Verification items for the finished model (mm, model axes). A direction names the side the tool comes from. Coordinates: 2 decimals unless noted, no trailing zeros. Order: outer loops, then holes, each group sorted by start corner. A loop starts at its lowest first (then second) coordinate and runs counter-clockwise, first axis right, second up. Notation, with made-up numbers: (81.5, 26.25) -> (105.5, 26.25) arc R14 ccw to (105.5, 35.25) -> close; hole circle Ø2 at (71, 81.25). An arc over 180 degrees is marked (long way). Write each question's results on one line, items separated by ' | '. Start each with the question number.
(1) Thickness scan on probe 1 along Y at (x, z) = (-5, 0); probe 2 along X at (y, z) = (2.35, 10); probe 3 along X at (y, z) = (-2, 1). Record the ranges inside material, lowest first. Write a range as [from, to].
(2) Cross-section at A-A on z = 10. Enter the section's corners in (x, y).
(3) Cross-section at D-D on y = -6.5. Enter the section's corners in (x, z), and give its area (3 significant figures).
(4) Draft check along X on faces 4 (the cylindrical face through (-9.51, 1.97, 9.87)), 5 (the cylindrical face through (-12.93, 2.03, -12.4)), 6 (the cylindrical face through (5, -8, 4)). Enter one of: +X half, -X half, draft (parallel to the pull), parting line (faces both ways), or undercut.
(5) Cross-section at C-C on y = 1. Enter the section's corners in (x, z), and give its area (3 significant figures).
(6) Set-up check for faces 1 (the flat face through (5, -2, 5)), 2 (the flat face through (7.5, -2.7, -0.1)), 3 (the flat face through (-5, -2, -5)): record each of +Z, -Z, +X, -X, +Y, -Y from which the full face is reachable in a straight line by a thin tool's end or side.
(7) Go/stop test with flat-tipped pins: pin 1 (8 mm diameter, centred on y = -4.5, z = -1.5, fed in from +X); pin 2 (3 mm diameter, centred on y = -3, z = -1, fed in from -X); pin 3 (1.5 mm diameter, centred on x = -10.5, y = -2.5, fed in from -Z); pin 4 (4 mm diameter, centred on x = 6, y = -2.5, fed in from +Z). Record where each tip stops, or that it passes through.
```python
from build123d import *

# Parameters (mm, degrees)
SKETCH1_W               = 27
SKETCH1_H               = 26
SKETCH1_R               = 1
BOSS_EXTRUDE1_DEPTH     = 4
SKETCH2_W               = 5
SKETCH2_H               = 10
BOSS_EXTRUDE2_DEPTH     = 10
FILLET1_R               = 5
CUT_EXTRUDE1_DEPTH      = 11
CUT_EXTRUDE1_DEPTH_BACK = 22
SKETCH4_R               = 2
FILLET2_R               = 2


with BuildPart() as part:
    # Sketch1 → Boss-Extrude1 (new body)
    with BuildSketch(Plane(origin=(0, 0, 0), x_dir=(1, 0, 0), z_dir=(0, 1, 0))):
        Rectangle(SKETCH1_W, SKETCH1_H)
        with Locations(Location((-10.5, 2.5, 0), (0, 0, 270))):
            Circle(SKETCH1_R, mode=Mode.SUBTRACT)
        with Locations(Location((-10.5, -10, 0), (0, 0, 270))):
            Circle(SKETCH1_R, mode=Mode.SUBTRACT)
        with Locations(Location((10.5, -10, 0), (0, 0, 270))):
            Circle(SKETCH1_R, mode=Mode.SUBTRACT)
        with Locations(Location((10.5, 2.5, 0), (0, 0, 270))):
            Circle(SKETCH1_R, mode=Mode.SUBTRACT)
    extrude(amount=BOSS_EXTRUDE1_DEPTH)

    # Sketch2 → Boss-Extrude2 (add)
    with BuildSketch(Plane.XZ):
        with Locations((-5, 0)):
            Rectangle(SKETCH2_W, SKETCH2_H)
        with Locations((5, 0)):
            Rectangle(SKETCH2_W, SKETCH2_H)
    extrude(amount=BOSS_EXTRUDE2_DEPTH)

    # Fillet1
    fillet1_edges = [part.edges().sort_by_distance(p)[0] for p in [
        (5, -10, 5),
        (5, -10, -5),
        (-5, -10, 5),
        (-5, -10, -5),
    ]]
    fillet(fillet1_edges, radius=FILLET1_R - 0.0001)  # a hair under: the kernel refuses the full size

    # Sketch4 → Cut-Extrude1 (cut, two sides: drawn at the far end of the back side and taken through both)
    with BuildSketch(Plane.ZY.offset(7.5).offset(-CUT_EXTRUDE1_DEPTH_BACK)):
        with Locations(Location((0, -5, 0), (0, 0, 180))):
            Circle(SKETCH4_R)
    extrude(amount=CUT_EXTRUDE1_DEPTH + CUT_EXTRUDE1_DEPTH_BACK, mode=Mode.SUBTRACT)

    # Fillet2
    fillet2_edges = [part.edges().sort_by_distance(p)[0] for p in [
        (-13.5, 2, 13),
        (-13.5, 2, -13),
        (13.5, 2, -13),
        (13.5, 2, 13),
    ]]
    fillet(fillet2_edges, radius=FILLET2_R)


solid = part.part
```
Results are:
1) probe 1: y = [-10, -7], [-3, 4] | probe 2: x = [-13.5, -11.5], [-9.5, 9.5], [11.5, 13.5] | probe 3: x = [-7.5, -2.5], [2.5, 7.5]
2) outline: (-13.5, 0) -> (-11.5, 0) -> (-11.5, 4) -> (-13.5, 4) -> close; (-9.5, 0) -> (9.5, 0) -> (9.5, 4) -> (-9.5, 4) -> close; (11.5, 0) -> (13.5, 0) -> (13.5, 4) -> (11.5, 4) -> close
3) outline: (-7.5, -4.77) -> (-2.5, -4.77) -> (-2.5, -1.32) -> (-7.5, -1.32) -> close; (-7.5, 1.32) -> (-2.5, 1.32) -> (-2.5, 4.77) -> (-7.5, 4.77) -> close; (2.5, -4.77) -> (7.5, -4.77) -> (7.5, -1.32) -> (2.5, -1.32) -> close; (2.5, 1.32) -> (7.5, 1.32) -> (7.5, 4.77) -> (2.5, 4.77) -> close | area: 68.9 mm2
4) face 4: undercut | face 5: -X half | face 6: draft
5) outline: (-13.5, -11) arc R2 ccw to (-11.5, -13) -> (11.5, -13) arc R2 ccw to (13.5, -11) -> (13.5, 11) arc R2 ccw to (11.5, 13) -> (-11.5, 13) arc R2 ccw to (-13.5, 11) -> close; hole circle Ø2 at (-10.5, -2.5); hole circle Ø2 at (-10.5, 10); hole circle Ø2 at (10.5, -2.5); hole circle Ø2 at (10.5, 10) | area: 686 mm2
6) face 1: +Z, +X, -X, -Y | face 2: +Z, -Z, +X, -Y | face 3: -Z, +X, -X, -Y
7) pin 1: stops at x = 7.5 | pin 2: stops at x = -7.5 | pin 3: passes through | pin 4: stops at z = 5
